Can you work these out from the drawing? Everything is in mm from the part's minimum corner. A direction names the side the tool comes from. Coordinates: 2 decimals unless noted, no trailing zeros. Loops run counter-clockwise (first coordinate to the right, second up) from the corner with the lowest first, then second, coordinate; pieces in that order, holes last. Notation, with made-up numbers: (33.5, -34) -> (73.5, -34) arc R15 ccw to (73.5, -20) -> close; hole circle Ø4 at (28, 32). An arc over 180 degrees is marked (long way). Use one line per item in the form item = value. Start each with the question number.
(1) Imagine slicing it at C-C (x = 61). List the corners of the cut face in (y, z) for me.
(2) I need wall thicknesses on line 1 (X direction, y = 36.85, z = 44); line 2 (X direction, y = 34, z = 39.5); line 3 (X direction, y = 28, z = 3.5). Which ranges of each line are inside material? Lowest first, please. Write a range as [from, to].
(3) On a 3-axis mill with a long thin cutter (end or side, diameter ignored), from which of +Z, -Z, +X, -X, +Y, -Y can I reach the whole of each face in a straight line? I mean the marked faces 1, 2 and 3. Say none if no direction works.
(4) Imagine slicing it at A-A (y = 17.5). List the corners of the cut face in (x, z) for me.
(5) I'm going to push flat-ended pins straight in: pin 1 (2 mm diameter, centred on x = 78, y = 27, fed in from -Z); pin 2 (4 mm diameter, centred on x = 63.5, z = 43, fed in from -Y); pin 3 (3 mm diameter, centred on x = 13, z = 27.5, fed in from +Y); pin 4 (15.5 mm diameter, centred on y = 28.5, z = 44, fed in from -X). Where does each tip first touch, or does it pass through?
(6) Imagine slicing it at B-B (z = 44). List the corners of the cut face in (x, y) for me.
(7) Thinking about a two-plate mould opening in Z: for the marked faces 4, 5 and 6, which applies, released by +Z, released by -Z, zero draft, split by the parting line, or undercut?
(8) Imagine slicing it at D-D (z = 34). List the corners of the cut face in (x, y) for me, plus the area to 3 significant figures.
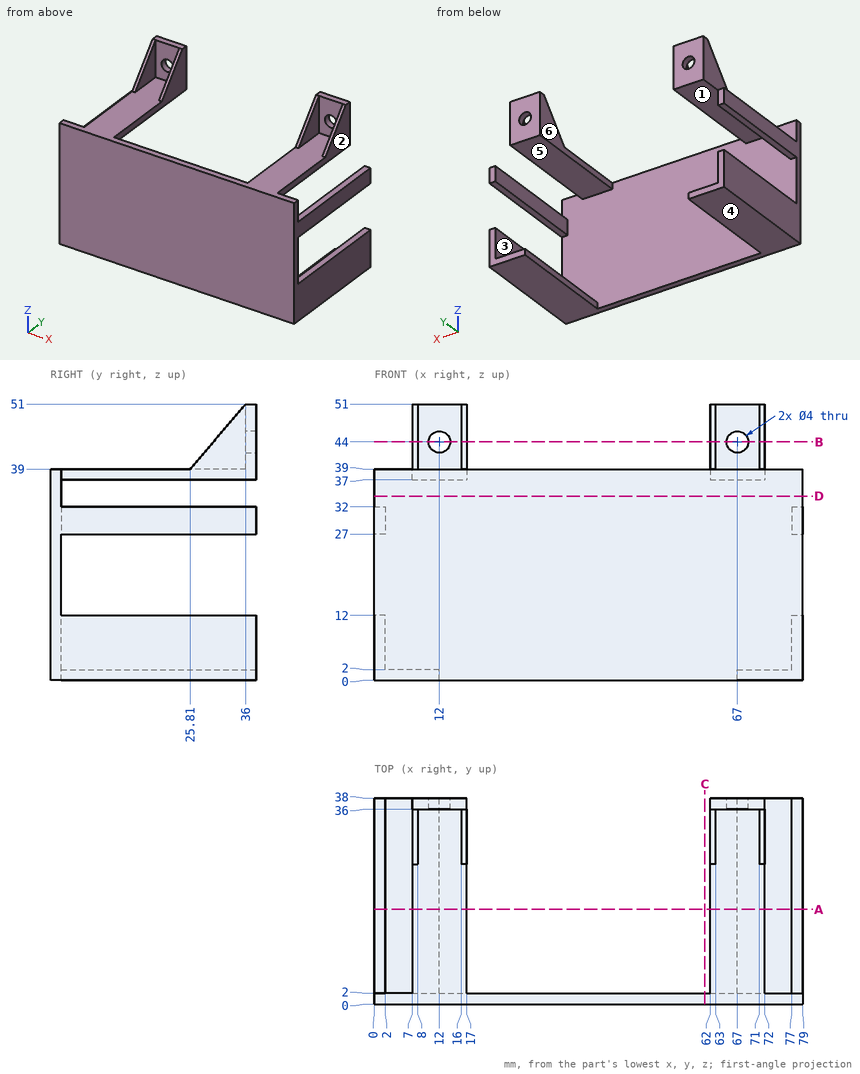
Worked out:
q1.outline = (0, 0) -> (2, 0) -> (2, 39) -> (0, 39) -> close
q2.line_1 = [7, 10], [14, 17], [62, 65], [69, 72]
q2.line_2 = [7, 8], [16, 17], [62, 63], [71, 72]
q2.line_3 = [0, 2], [77, 79]
q3.face_1 = +X, -X, +Y
q3.face_2 = +Z, +X, +Y
q3.face_3 = +Z, +Y
q4.outline = (0, 0) -> (12, 0) -> (12, 2) -> (2, 2) -> (2, 12) -> (0, 12) -> close; (0, 27) -> (2, 27) -> (2, 32) -> (0, 32) -> close; (7, 37) -> (17, 37) -> (17, 39) -> (7, 39) -> close; (62, 37) -> (72, 37) -> (72, 39) -> (62, 39) -> close; (67, 0) -> (79, 0) -> (79, 12) -> (77, 12) -> (77, 2) -> (67, 2) -> close; (77, 27) -> (79, 27) -> (79, 32) -> (77, 32) -> close
q5.pin_1 = 0
q5.pin_2 = 27.56
q5.pin_3 = 2
q5.pin_4 = 7
q6.outline = (7, 30.06) -> (8, 30.06) -> (8, 36) -> (10, 36) -> (10, 38) -> (7, 38) -> close; (14, 36) -> (16, 36) -> (16, 30.06) -> (17, 30.06) -> (17, 38) -> (14, 38) -> close; (62, 30.06) -> (63, 30.06) -> (63, 36) -> (65, 36) -> (65, 38) -> (62, 38) -> close; (69, 36) -> (71, 36) -> (71, 30.06) -> (72, 30.06) -> (72, 38) -> (69, 38) -> close
q7.face_4 = released by -Z
q7.face_5 = undercut
q7.face_6 = zero draft
q8.outline = (0, 0) -> (79, 0) -> (79, 2) -> (0, 2) -> close
q8.area = 158 mm2
